Read the model definition and answer for the solid it produces. Units are mm, in the model's axes. Round coordinates to 2 decimals unless told otherwise and drop trailing zeros. Write each loop counter-clockwise with the first axis right and the second up, starting at its lowest first coordinate (ties: lowest second). Pieces come first, ordered by that corner, then holes. Notation, with made-up numbers: (5, 49.5) -> (41, 49.5) arc R19 cw to (41, 69.5) -> close; hole circle Ø9 at (88.5, -3.75). An arc over 180 degrees is marked (long way). Return JSON: item names as keys, results as strings. Group by question number.
(1) A cutting plane is placed at B-B on x = 76. Give the vertices of the cut face in (y, z).
(2) A cutting plane is placed at D-D on x = -350. Give the vertices of the cut face in (y, z), then the cut area to 3 significant figures.
(3) Given pin 1 (1 mm diameter, centred on x = -392.5, y = 71, fed in from -Z); pin 2 (21 mm diameter, centred on x = 362, z = 561, fed in from -Y); pin 3 (18 mm diameter, centred on y = 73.5, z = -841, fed in from -X), each flat-ended and moving along its own axis, determine where each tip first touches the part or whether it passes through.
(4) A cutting plane is placed at A-A on z = 39. Give the vertices of the cut face in (x, y), then the cut area to 4 significant figures.
(5) Straight lines are drawn through the part: line 1 (Z direction, x = -74, y = 34.5); line 2 (Y direction, x = -179.5, z = 402.5); line 3 (X direction, y = 57, z = 744). For each, find the intervals that lie inside material, in ascending order.
(6) A cutting plane is placed at C-C on z = -479. Give the vertices of the cut face in (x, y).
```python
from build123d import *

# Parameters (mm, degrees)
BOSS_EXTRUDE1_DEPTH     = 150
SKETCH2_W               = 400
SKETCH2_H               = 65
CUT_EXTRUDE1_DEPTH      = 1
CUT_EXTRUDE1_DEPTH_BACK = 1501
SKETCH3_W               = 600
SKETCH3_H               = 65
CUT_EXTRUDE2_DEPTH      = 130
SKETCH4_R               = 5
BOSS_EXTRUDE2_DEPTH     = 150
SKETCH6_W               = 55
SKETCH6_H               = 60
CUT_EXTRUDE4_DEPTH      = 200
CUT_EXTRUDE5_DEPTH      = 130
SKETCH8_W               = 1230
SKETCH8_H               = 55
CUT_EXTRUDE6_DEPTH      = 600
SKETCH9_W               = 180
SKETCH9_H               = 135
CUT_EXTRUDE7_DEPTH      = 120


with BuildPart() as part:
    # Sketch1 → Boss-Extrude1 (new body)
    with BuildSketch(Plane(origin=(0, 0, 0), x_dir=(1, 0, 0), z_dir=(0, 1, 0))):
        with BuildLine():
            Line((-550, 1000), (-225, 1000))
            Line((-225, 1000), (225, 1000))
            Line((225, 1000), (550, 1000))
            ThreePointArc((550, 1000), (691.421356237, 941.421356237), (750, 800))
            Line((750, 800), (750, -800))
            ThreePointArc((750, -800), (691.421356237, -941.421356237), (550, -1000))
            Line((550, -1000), (-550, -1000))
            ThreePointArc((-550, -1000), (-691.421356237, -941.421356237), (-750, -800))
            Line((-750, -800), (-750, 800))
            ThreePointArc((-750, 800), (-691.421356237, 941.421356237), (-550, 1000))
        make_face()
    extrude(amount=BOSS_EXTRUDE1_DEPTH)

    # Sketch2 → Cut-Extrude1 (cut, two sides)
    with BuildSketch(Plane(origin=(750, 0, 0), x_dir=(0, 0, -1), z_dir=(1, 0, 0))) as cut_extrude1_sk:
        with Locations((0, 42.5)):
            Rectangle(SKETCH2_W, SKETCH2_H)
    extrude(amount=CUT_EXTRUDE1_DEPTH, mode=Mode.SUBTRACT)
    extrude(cut_extrude1_sk.sketch, amount=-CUT_EXTRUDE1_DEPTH_BACK, mode=Mode.SUBTRACT)

    # Sketch3 → Cut-Extrude2 (cut)
    with BuildSketch(Plane(origin=(750, 0, 0), x_dir=(0, 0, -1), z_dir=(1, 0, 0))):
        with Locations((500, 42.5)):
            Rectangle(SKETCH3_W, SKETCH3_H)
        with Locations((-500, 42.5)):
            Rectangle(SKETCH3_W, SKETCH3_H)
    cut_extrude2 = extrude(amount=-CUT_EXTRUDE2_DEPTH, mode=Mode.SUBTRACT)

    # Mirror1: Cut-Extrude2 across plane
    add(cut_extrude2.mirror(Plane(origin=(0, 0, 0), x_dir=(0, 0, 1), z_dir=(1, 0, 0))), mode=Mode.SUBTRACT)

    # Sketch4 → Boss-Extrude2 (add)
    with BuildSketch(Plane(origin=(0, 150, 0), x_dir=(1, 0, 0), z_dir=(0, 1, 0))):
        with Locations((-670, 100)):
            Circle(SKETCH4_R)
        with Locations((-670, -100)):
            Circle(SKETCH4_R)
    boss_extrude2 = extrude(amount=-BOSS_EXTRUDE2_DEPTH)

    # Mirror2: Boss-Extrude2 across plane
    add(boss_extrude2.mirror(Plane(origin=(0, 0, 0), x_dir=(0, 0, 1), z_dir=(1, 0, 0))))

    # Sketch6 → Cut-Extrude4 (cut)
    with BuildSketch(Plane(origin=(0, 0, -1000), x_dir=(-1, 0, 0), z_dir=(0, 0, -1))):
        with Locations((-350, 75)):
            Rectangle(SKETCH6_W, SKETCH6_H)
        with Locations((350, 75)):
            Rectangle(SKETCH6_W, SKETCH6_H)
    extrude(amount=-CUT_EXTRUDE4_DEPTH, mode=Mode.SUBTRACT)

    # Sketch7 → Cut-Extrude5 (cut)
    with BuildSketch(Plane.XZ):
        with BuildLine():
            Line((385, 480), (385, 600))
            ThreePointArc((385, 600), (350, 635), (315, 600))
            Line((315, 600), (315, 480))
            ThreePointArc((315, 480), (350, 445), (385, 480))
        make_face()
        with BuildLine():
            Line((-315, 480), (-315, 600))
            ThreePointArc((-315, 600), (-350, 635), (-385, 600))
            Line((-385, 600), (-385, 480))
            ThreePointArc((-385, 480), (-350, 445), (-315, 480))
        make_face()
    extrude(amount=-CUT_EXTRUDE5_DEPTH, mode=Mode.SUBTRACT)

    # Sketch8 → Cut-Extrude6 (cut)
    with BuildSketch(Plane(origin=(0, 0, 200), x_dir=(-1, 0, 0), z_dir=(0, 0, -1))):
        with Locations((0, 42.5)):
            Rectangle(SKETCH8_W, SKETCH8_H)
    extrude(amount=-CUT_EXTRUDE6_DEPTH, mode=Mode.SUBTRACT)

    # Sketch9 → Cut-Extrude7 (cut)
    with BuildSketch(Plane(origin=(0, 0, -1000), x_dir=(-1, 0, 0), z_dir=(0, 0, -1))):
        with Locations((-350, 75)):
            Rectangle(SKETCH9_W, SKETCH9_H)
        with Locations((350, 75)):
            Rectangle(SKETCH9_W, SKETCH9_H)
    extrude(amount=-CUT_EXTRUDE7_DEPTH, mode=Mode.SUBTRACT)


solid = part.part
```
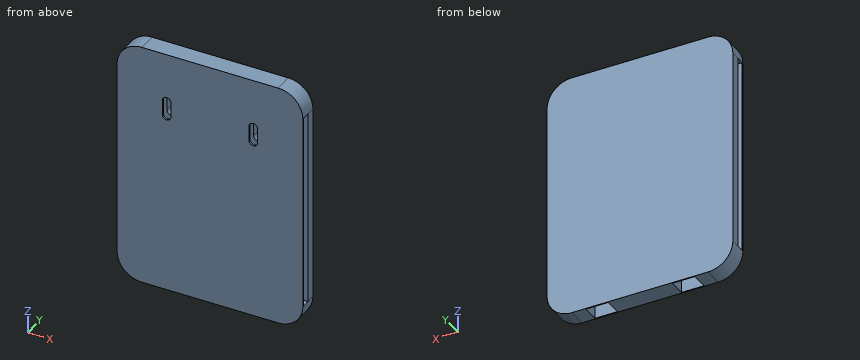
Checks:
{
 "1": {"outline": "(0, -1000) -> (150, -1000) -> (150, 1000) -> (0, 1000) -> close; hole (10, -200) -> (75, -200) -> (75, 200) -> (70, 200) -> (70, 800) -> (15, 800) -> (15, 200) -> (10, 200) -> close"},
 "2": {"outline": "(0, -1000) -> (7.5, -1000) -> (7.5, -880) -> (45, -880) -> (45, -800) -> (105, -800) -> (105, -880) -> (142.5, -880) -> (142.5, -1000) -> (150, -1000) -> (150, 1000) -> (0, 1000) -> (0, 635) -> (15, 635) -> (15, 800) -> (70, 800) -> (70, 635) -> (130, 635) -> (130, 445) -> (70, 445) -> (70, 200) -> (75, 200) -> (75, -200) -> (10, -200) -> (10, 200) -> (15, 200) -> (15, 445) -> (0, 445) -> close", "area": "206,000 mm^2"},
 "3": {"pin 1": "stops at z = -880", "pin 2": "stops at y = 130", "pin 3": "stops at x = -747.42"},
 "4": {"outline": "(-750, 0) -> (750, 0) -> (750, 10) -> (-750, 10) -> close; (-750, 75) -> (750, 75) -> (750, 150) -> (-750, 150) -> close", "area": "127,500 mm^2"},
 "5": {"line 1": "z = -1000 to -200, 800 to 1000", "line 2": "y = 0 to 15, 70 to 150", "line 3": "x = -620 to -615, 615 to 620"},
 "6": {"outline": "(-750, 0) -> (750, 0) -> (750, 10) -> (620, 10) -> (620, 75) -> (750, 75) -> (750, 150) -> (-750, 150) -> (-750, 75) -> (-620, 75) -> (-620, 10) -> (-750, 10) -> close"}
}
